from build123d import *

# Parameters (mm, degrees)
SKETCH2_R           = 76.2
SKETCH2_R_2         = 3.302
SKETCH2_R_3         = 4.7625
BOSS_EXTRUDE1_DEPTH = 3.175
CUT_EXTRUDE1_DEPTH  = 6.35
SKETCH4_R           = 1.7526
CUT_EXTRUDE2_DEPTH  = 18.034
CIRPATTERN1_COUNT   = 13


with BuildPart() as part:
    # Sketch2 → Boss-Extrude1 (new, symmetric)
    with BuildSketch(Plane.XY):
        Circle(SKETCH2_R)
        with Locations((-50.8, 0)):
            Circle(SKETCH2_R_2, mode=Mode.SUBTRACT)
        with Locations((50.8, 0)):
            Circle(SKETCH2_R_2, mode=Mode.SUBTRACT)
        with Locations((0, 23.8125)):
            Circle(SKETCH2_R_3, mode=Mode.SUBTRACT)
        with Locations((0, -23.8125)):
            Circle(SKETCH2_R_3, mode=Mode.SUBTRACT)
    extrude(amount=BOSS_EXTRUDE1_DEPTH, both=True)

    # Sketch3 → Cut-Extrude1 (cut)
    with BuildSketch(Plane(origin=(0, 0, -3.175), x_dir=(-1, 0, 0), z_dir=(0, 0, -1))):
        with BuildLine():
            Line((-27.94, -11.43), (-22.86, -11.43))
            ThreePointArc((-22.86, -11.43), (-19.05, -15.24), (-22.86, -19.05))
            Line((-22.86, -19.05), (-27.94, -19.05))
            ThreePointArc((-27.94, -19.05), (-31.75, -15.24), (-27.94, -11.43))
        make_face()
    cut_extrude1 = extrude(amount=-CUT_EXTRUDE1_DEPTH, mode=Mode.SUBTRACT)

    # Mirror1: Cut-Extrude1 across plane
    add(cut_extrude1.mirror(Plane(origin=(0, 0, 0), x_dir=(0, 0, 1), z_dir=(1, 0, 0))), mode=Mode.SUBTRACT)

    # Sketch4 → Cut-Extrude2 (cut)
    with BuildSketch(Plane.XY.offset(3.175)):
        with Locations((-68.326, 0)):
            Circle(SKETCH4_R)
    cut_extrude2 = extrude(amount=-CUT_EXTRUDE2_DEPTH, mode=Mode.SUBTRACT)

    # CirPattern1: Cut-Extrude2 ×13 about axis
    cirpattern1_axis = Axis((0, 0, 0), (0, 0, 1))
    for i in range(1, CIRPATTERN1_COUNT):
        add(cut_extrude2.rotate(cirpattern1_axis, i * 360 / CIRPATTERN1_COUNT), mode=Mode.SUBTRACT)


solid = part.part
Could you check a few things on this model? Use its own coordinates, in mm. Round coordinates to 2 decimals unless told otherwise and drop trailing zeros. Write each loop counter-clockwise with the first axis right and the second up, starting at its lowest first coordinate (ties: lowest second). Pieces come first, ordered by that corner, then holes. Notation, with made-up numbers: (72, 40) - (98, 40) arc R31 ccw to (98, 64) - close; hole circle Ø10 at (51.25, -37.5). An arc over 180 degrees is marked (long way). Use a Markdown table: item, result.
Q1. Please list where these lines run through material, in increasing order: L1, parallel to Y at x = 0, z = -0.75 (3 decimals); L2, parallel to Y at x = -3, z = -0.5; L3, parallel to X at y = 1.5, z = 0.25.
Output values:
| item | result |
|---|---|
| L1 | -76.2 to -28.575, -19.05 to 19.05, 28.575 to 76.2 |
| L2 | -76.14 to -27.51, -20.11 to 20.11, 27.51 to 76.14 |
| L3 | -76.19 to -69.23, -67.42 to -53.74, -47.86 to 47.86, 53.74 to 76.19 |
Q2. For pin 1 (2 mm diameter, centred on y = 47, z = 1.5, fed in from +X); pin 2 (2 mm diameter, centred on x = -8.24, y = -67.83, fed in from +Z); pin 3 (3 mm diameter, centred on x = -55.5, z = -2.5, fed in from +Y); pin 4 (2.5 mm diameter, centred on x = -25.5, z = -1, fed in from -Y), each with a flat end and sliding along its axis, tell me the tip position at first contact or that it passes through.
Output values:
| item | result |
|---|---|
| pin 1 | x = 60.75 |
| pin 2 | through |
| pin 3 | y = 53.76 |
| pin 4 | y = -72.24 |
Q3. I want a section at A-A (y = 0). List the corners of the cut face in (x, z) for me (3 decimals), plus the area to 3 significant figures.
Output values:
| item | result |
|---|---|
| outline | (-76.2, -3.175) - (-70.079, -3.175) - (-70.079, 3.175) - (-76.2, 3.175) - close; (-66.573, -3.175) - (-54.102, -3.175) - (-54.102, 3.175) - (-66.573, 3.175) - close; (-47.498, -3.175) - (47.498, -3.175) - (47.498, 3.175) - (-47.498, 3.175) - close; (54.102, -3.175) - (76.2, -3.175) - (76.2, 3.175) - (54.102, 3.175) - close |
| area | 862 mm2 |
Q4. I want a section at C-C (x = 0). List the corners of the cut face in (y, z) for me (3 decimals).
Output values:
| item | result |
|---|---|
| outline | (-76.2, -3.175) - (-28.575, -3.175) - (-28.575, 3.175) - (-76.2, 3.175) - close; (-19.05, -3.175) - (19.05, -3.175) - (19.05, 3.175) - (-19.05, 3.175) - close; (28.575, -3.175) - (76.2, -3.175) - (76.2, 3.175) - (28.575, 3.175) - close |
Q5. I want a section at D-D (z = 0.75). Count the separate pieces of the cut face and the enclosed holes in it, plus the area to 3 significant figures.
Output values:
| item | result |
|---|---|
| separate pieces | 1 |
| enclosed holes | 19 |
| area | 17,700 mm2 |
Q6. I want a section at B-B (x = -50.8). List the corners of the cut face in (y, z) for me (3 decimals).
Output values:
| item | result |
|---|---|
| outline | (-56.796, -3.175) - (-3.302, -3.175) - (-3.302, 3.175) - (-56.796, 3.175) - close; (3.302, -3.175) - (56.796, -3.175) - (56.796, 3.175) - (3.302, 3.175) - close |
